Answer from the drawing. Dimensions are ordinates in mm from the lowest x, y and z of the part. A direction names the side the tool comes from. Coordinates: 2 decimals unless noted, no trailing zeros. Loops run counter-clockwise (first coordinate to the right, second up) from the corner with the lowest first, then second, coordinate; pieces in that order, holes last. Notation, with made-up numbers: M -11,5.25 L 47,5.25 A20 ccw 47,21.25 Z; hole C 0,9 d11. An arc over 180 degrees is marked long. Answer as CSV lines item,"result". Start each with the question number.
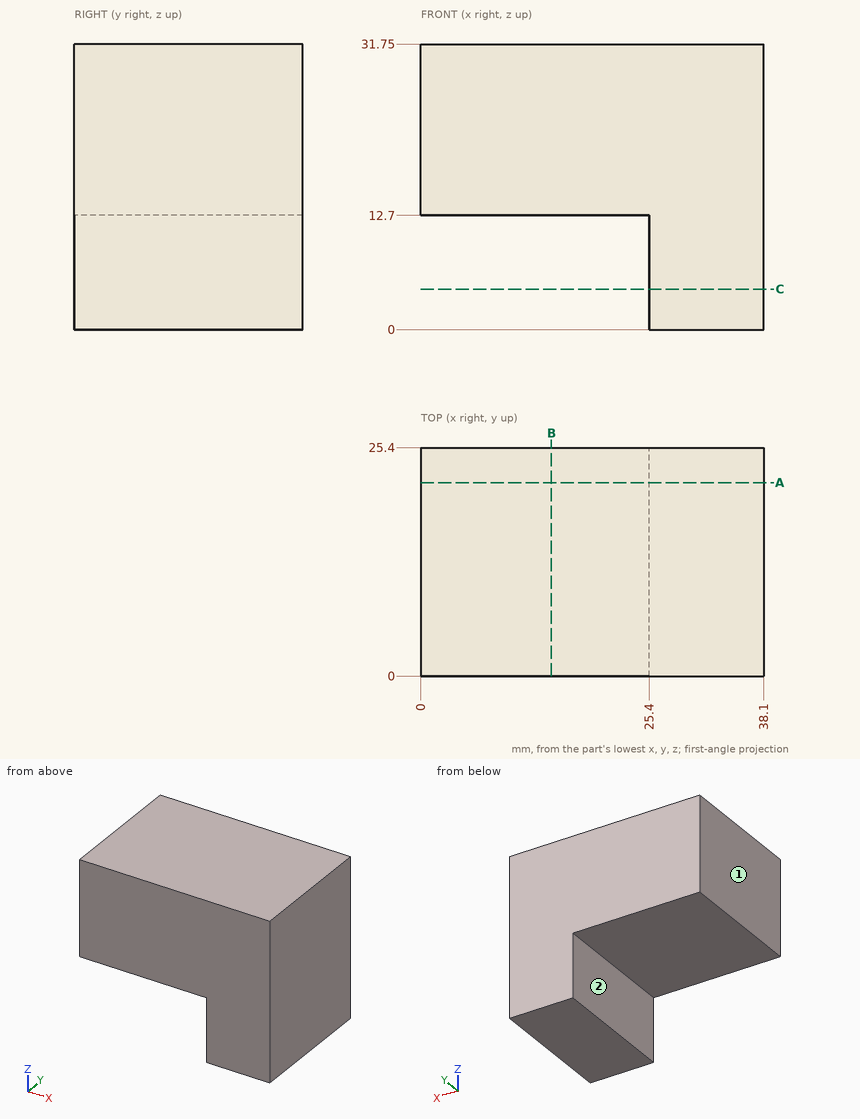
Item 1: For the marked faces 1 and 2, determine the directions among +Z, -Z, +X, -X, +Y, -Y from which every point of the face is accessible in a straight line to the end or side of a thin tool.
Item 2: Section B-B on x = 14.5 is taken. Determine the outline of the cut face in (y, z).
Item 3: Section C-C on z = 4.5 is taken. Determine the outline of the cut face in (x, y), then the cut area to 3 significant figures.
Item 4: Section A-A on y = 21.5 is taken. Determine the outline of the cut face in (x, z).
Item 5: Each of these flat-tipped pins is pushed along its axis until it touches: P1, Ø14, axis at y = 13, z = 6, coming from the -X side; P2, Ø1, axis at y = 9, z = 5.5, coming from the -X side. Where does it stop, or does it pass through?
Item 6: Consider line 1 (Z direction, x = 20, y = 10.5); line 2 (X direction, y = 12.75, z = 8.5). Determine where each line is inside the solid, lowest interval first.
Results are:
1,face 1,"+Z, -Z, -X, +Y, -Y"
1,face 2,"-Z, -X, +Y, -Y"
2,outline,"M 0,12.7 L 25.4,12.7 L 25.4,31.75 L 0,31.75 Z"
3,outline,"M 25.4,0 L 38.1,0 L 38.1,25.4 L 25.4,25.4 Z"
3,area,"323 mm²"
4,outline,"M 0,12.7 L 25.4,12.7 L 25.4,0 L 38.1,0 L 38.1,31.75 L 0,31.75 Z"
5,P1,"x = 0"
5,P2,"x = 25.4"
6,line 1,"12.7 to 31.75"
6,line 2,"25.4 to 38.1"
